The listing builds one solid part. Answer for the finished solid, in the listing's coordinates (mm). A direction names the side the tool comes from. Coordinates: 2 decimals unless noted, no trailing zeros. Loops run counter-clockwise (first coordinate to the right, second up) from the corner with the lowest first, then second, coordinate; pieces in that order, holes last. Notation, with made-up numbers: (5, 18.5) - (23, 18.5) arc R24 cw to (23, 33.5) - close; hole circle Ø9 at (6.25, -28.5). An arc over 180 degrees is marked (long way). Return JSON: item names as keys, results as strings. Group by question number.
1. Find the intervals of material crossed by line 1 along Z through (x, y) = (3.75, -3.5); line 2 along Z through (x, y) = (-2.75, 8.5); line 3 along Y through (x, z) = (-2, 4.8), in increasing order.
2. Which of the six approach directions +Z, -Z, +X, -X, +Y, -Y give full straight-line access (tool end or side, diameter ignored) to faces 1 (the face through (0, 0, 0)), 2 (the face through (-9.137, 3.629, 4.853)), 3 (the face through (2.3, -2.3, 4.1))?
3. Section B-B (z = 2.7) is taken. Write down the section's boundary in (x, y).
4. Each of these flat-tipped pins is pushed along its axis until it touches: P1, Ø0.6, axis at y = 3.5, z = 5, coming from the +X side; P2, Ø0.6, axis at x = -1.5, z = 5, coming from the -Y side; P3, Ø5, axis at x = -4, y = 6, coming from the -Z side. Where does it stop, or does it pass through?
5. Section D-D (y = -8) is taken. Write down the section's boundary in (x, z), and give its area (3 significant figures).
6. The mould has two halves that part along X. Classify faces 4 (the face through (-2.38, -10.74, 4.59)), 5 (the face through (7, 1, 4.6)), 6 (the face through (3, 0, 4.6)), 7 (the face through (0, 0, 5.1)): pulls with the +X half, pulls with the -X half, needs draft (parallel to the pull), parting line crosses it, or undercut.
7. Section C-C (x = 6.5) is taken. Write down the section's boundary in (y, z).
8. Section A-A (x = 0) is taken. Write down the section's boundary in (y, z), and give its area (3 significant figures).
```python
from build123d import *

# Parameters (mm, degrees)
F0_R     = 2.45
F1_DEPTH = 3.6
F2_R     = 3
F2_R_2   = 2.45
F3_DEPTH = 0.5
F4_R     = 11
F4_R_2   = 3
F5_DEPTH = 1
F6_W     = 1.534777
F6_H     = 2.504423
F7_DEPTH = 0.5


with BuildPart() as f1:
    # F0 (on Top) → F1 (new body)
    with BuildSketch(Plane.XY):
        Circle(F0_R)
    extrude(amount=F1_DEPTH)

    # F2 (on face) → F3 (join)
    with BuildSketch(Plane.XY.offset(3.6)):
        Circle(F2_R)
        Circle(F2_R_2, mode=Mode.SUBTRACT)
        Circle(F2_R_2)
    extrude(amount=F3_DEPTH)

    # F4 (on face) → F5 (join)
    with BuildSketch(Plane.XY.offset(4.1)):
        Circle(F4_R)
        Circle(F4_R_2, mode=Mode.SUBTRACT)
        Circle(F4_R_2)
    extrude(amount=F5_DEPTH)

    # F6 (on face) → F7 (cut)
    with BuildSketch(Plane.XY.offset(5.1)):
        Polygon((-9.839244, -4.300933), (-8.030824, -4.300933), (-8.030824, -1.475277), (-6.496047, -1.475277), (-6.496047, -4.300933), (-4.693576, -4.300933), (-4.693576, 4.300958), (-8.453185, 4.300958), (-9.839244, 2.938695), align=None)
        with Locations((-7.263435, 1.41284)):
            Rectangle(F6_W, F6_H, mode=Mode.SUBTRACT)
        Polygon((-0.39263, 2.665052), (1.231378, 2.665052), (1.231378, 4.300958), (-3.890495, 4.300958), (-3.890495, 2.665052), (-2.206999, 2.665052), (-2.206999, -4.300933), (-0.39263, -4.300933), align=None)
        Polygon((4.955295, -4.300933), (4.955295, -2.670976), (4.36042, -2.670976), (4.36042, 2.671001), (4.955295, 2.671001), (4.955295, 4.300958), (1.963075, 4.300958), (1.963075, 2.671001), (2.557949, 2.671001), (2.557949, -2.670976), (1.963075, -2.670976), (1.963075, -4.300933), align=None)
        Polygon((7.531104, -4.300933), (7.531104, -0.600811), (9.660756, -0.600811), (9.660756, 1.005351), (7.531104, 1.005351), (7.531104, 2.665052), (9.839219, 2.665052), (9.839219, 4.300958), (6.918383, 4.300958), (5.728633, 3.111209), (5.728633, -4.300933), align=None)
    extrude(amount=-F7_DEPTH, mode=Mode.SUBTRACT)


solid = f1.part
```
The answers:
{
 "1": {"line 1": "z = 4.1 to 4.6", "line 2": "z = 4.1 to 5.1", "line 3": "y = -10.82 to -4.3, 4.3 to 10.82"},
 "2": {"face 1": "-Z, +X, -X, +Y, -Y", "face 2": "+Z", "face 3": "-Z"},
 "3": {"outline": "circle Ø4.9 at (0, 0)"},
 "4": {"P1": "stops at x = 10.52", "P2": "stops at y = -10.93", "P3": "stops at z = 4.1"},
 "5": {"outline": "(-7.55, 4.1) - (7.55, 4.1) - (7.55, 5.1) - (-7.55, 5.1) - close", "area": "15.1 mm2"},
 "6": {"face 4": "parting line crosses it", "face 5": "undercut", "face 6": "undercut", "face 7": "needs draft"},
 "7": {"outline": "(-8.87, 4.1) - (8.87, 4.1) - (8.87, 5.1) - (3.88, 5.1) - (3.88, 4.6) - (-4.3, 4.6) - (-4.3, 5.1) - (-8.87, 5.1) - close"},
 "8": {"outline": "(-11, 4.1) - (-3, 4.1) - (-3, 3.6) - (-2.45, 3.6) - (-2.45, 0) - (2.45, 0) - (2.45, 3.6) - (3, 3.6) - (3, 4.1) - (11, 4.1) - (11, 5.1) - (4.3, 5.1) - (4.3, 4.6) - (2.67, 4.6) - (2.67, 5.1) - (-11, 5.1) - close", "area": "41.8 mm2"}
}
